Check sheet for the drawn part. Datum: minimum x, y, z corner. Units: mm. A direction names the side the tool comes from. Round coordinates to 2 decimals unless told otherwise and drop trailing zeros. Loops run counter-clockwise (first coordinate to the right, second up) from the corner with the lowest first, then second, coordinate; pieces in that order, holes last. Notation, with made-up numbers: (-6.5, 75) -> (-2.5, 75) arc R26 cw to (-2.5, 92) -> close; hole circle Ø7 at (68, -35.5). An arc over 180 degrees is marked (long way). Return JSON: item names as keys, results as strings.
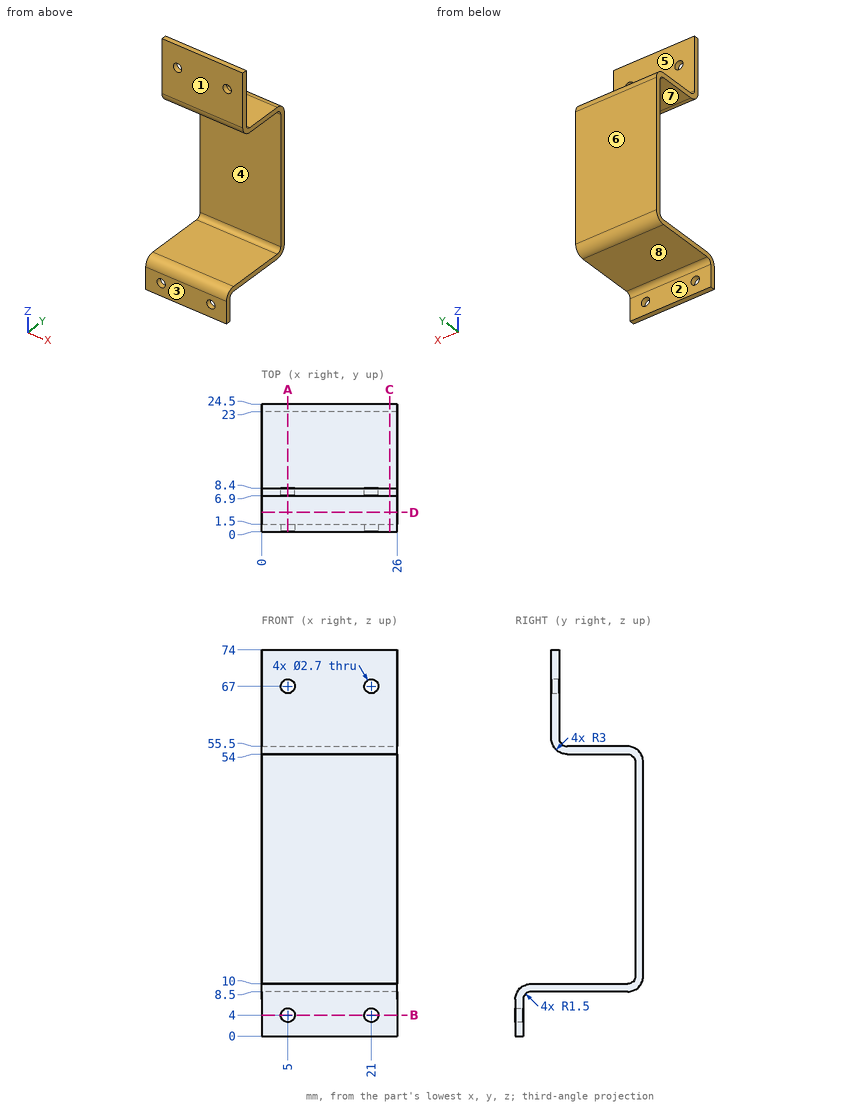
Q1. Tool access check on the marked faces 1, 2, 3, 4 and 5. Record the directions out of +Z, -Z, +X, -X, +Y, -Y that give a thin tool (end or side, any length) a straight path to the whole face; none if there is none.
Results list:
{"face 1": "+Z, +X, -X, -Y", "face 2": "-Z, +X, -X, +Y", "face 3": "+Z, -Z, +X, -X, -Y", "face 4": "+X, -X, -Y", "face 5": "+Z, +X, -X, +Y"}
Q2. Section check A-A (x = 5). Record the boundary of the cut face in (y, z).
Results list:
{"outline": "(0, 0) -> (1.5, 0) -> (1.5, 2.65) -> (0, 2.65) -> close; (0, 5.35) -> (1.5, 5.35) -> (1.5, 7) arc R1.5 cw to (3, 8.5) -> (21.5, 8.5) arc R3 ccw to (24.5, 11.5) -> (24.5, 52.5) arc R3 ccw to (21.5, 55.5) -> (9.9, 55.5) arc R1.5 cw to (8.4, 57) -> (8.4, 65.65) -> (6.9, 65.65) -> (6.9, 57) arc R3 ccw to (9.9, 54) -> (21.5, 54) arc R1.5 cw to (23, 52.5) -> (23, 11.5) arc R1.5 cw to (21.5, 10) -> (3, 10) arc R3 ccw to (0, 7) -> close; (6.9, 68.35) -> (8.4, 68.35) -> (8.4, 74) -> (6.9, 74) -> close"}
Q3. Section check B-B (z = 4). Record the boundary of the cut face in (x, y), then the cut area to 3 significant figures.
Results list:
{"outline": "(0, 0) -> (3.65, 0) -> (3.65, 1.5) -> (0, 1.5) -> close; (6.35, 0) -> (19.65, 0) -> (19.65, 1.5) -> (6.35, 1.5) -> close; (22.35, 0) -> (26, 0) -> (26, 1.5) -> (22.35, 1.5) -> close", "area": "30.9 mm^2"}
Q4. Material ranges on line 1 (X direction, y = 8.1, z = 67); line 2 (Z direction, x = 9.5, y = 12.75); line 3 (Y direction, x = 21.75, z = 30), recorded low to high.
Results list:
{"line 1": "0 to 3.65, 6.35 to 19.65, 22.35 to 26", "line 2": "8.5 to 10, 54 to 55.5", "line 3": "23 to 24.5"}
Q5. Draft check along Z on the marked faces 6, 7 and 8. Enter one of: released by +Z, released by -Z, zero draft, split by the parting line, or undercut.
Results list:
{"face 6": "zero draft", "face 7": "undercut", "face 8": "released by -Z"}
Q6. Go/stop test with flat-tipped pins: pin 1 (5 mm diameter, centred on x = 6, y = 11, fed in from -Z); pin 2 (2.5 mm diameter, centred on x = 5, z = 67, fed in from -Y); pin 3 (6 mm diameter, centred on x = 18, y = 14, fed in from +Z); pin 4 (8.5 mm diameter, centred on x = 13.5, z = 67.5, fed in from +Y). Record where each tip stops, or that it passes through.
Results list:
{"pin 1": "z = 8.5", "pin 2": "through", "pin 3": "z = 55.5", "pin 4": "y = 8.4"}
Q7. Section check D-D (y = 3.75). Record the boundary of the cut face in (x, z), then the cut area to 3 significant figures.
Results list:
{"outline": "(0, 8.5) -> (26, 8.5) -> (26, 10) -> (0, 10) -> close", "area": "39.0 mm^2"}
Q8. Section check C-C (x = 24.5). Record the boundary of the cut face in (y, z), then the cut area to 3 significant figures.
Results list:
{"outline": "(0, 0) -> (1.5, 0) -> (1.5, 7) arc R1.5 cw to (3, 8.5) -> (21.5, 8.5) arc R3 ccw to (24.5, 11.5) -> (24.5, 52.5) arc R3 ccw to (21.5, 55.5) -> (9.9, 55.5) arc R1.5 cw to (8.4, 57) -> (8.4, 74) -> (6.9, 74) -> (6.9, 57) arc R3 ccw to (9.9, 54) -> (21.5, 54) arc R1.5 cw to (23, 52.5) -> (23, 11.5) arc R1.5 cw to (21.5, 10) -> (3, 10) arc R3 ccw to (0, 7) -> close", "area": "164 mm^2"}
